from build123d import *

# Parameters (mm, degrees)
SKETCH_1_W      = 55
SKETCH_1_H      = 25
EXTRUDE_1_DEPTH = 1
FILLET_1_R      = 2


with BuildPart() as part:
    # Эскиз1 → Бобышка-Вытянуть1 (new body)
    with BuildSketch(Plane(origin=(0, 0, 0), x_dir=(1, 0, 0), z_dir=(0, 1, 0))):
        with Locations((-2.718269759, 0.212657213)):
            Rectangle(SKETCH_1_W, SKETCH_1_H)
        with BuildLine():
            Line((-18.218269759, 2.212657213), (-18.218269759, -1.787342787))
            ThreePointArc((-18.218269759, -1.787342787), (-20.218269759, -3.787342787), (-22.218269759, -1.787342787))
            Line((-22.218269759, -1.787342787), (-22.218269759, 2.212657213))
            ThreePointArc((-22.218269759, 2.212657213), (-20.218269759, 4.212657213), (-18.218269759, 2.212657213))
        make_face(mode=Mode.SUBTRACT)
        with BuildLine():
            Line((12.781730241, 2.212657213), (12.781730241, -1.787342787))
            ThreePointArc((12.781730241, -1.787342787), (14.781730241, -3.787342787), (16.781730241, -1.787342787))
            Line((16.781730241, -1.787342787), (16.781730241, 2.212657213))
            ThreePointArc((16.781730241, 2.212657213), (14.781730241, 4.212657213), (12.781730241, 2.212657213))
        make_face(mode=Mode.SUBTRACT)
    extrude(amount=EXTRUDE_1_DEPTH)

    # Скругление1
    fillet_1_edges = [part.edges().sort_by_distance(p)[0] for p in [
        (24.781730241, 0.5, 12.287342787),
        (-30.218269759, 0.5, 12.287342787),
        (-30.218269759, 0.5, -12.712657213),
        (24.781730241, 0.5, -12.712657213),
    ]]
    fillet(fillet_1_edges, radius=FILLET_1_R)


solid = part.part
Model file for the job. Use its own axes, mm. A direction names the side the tool comes from. Round coordinates to 2 decimals unless told otherwise and drop trailing zeros. Order: outer loops, then holes, each group sorted by start corner. A loop starts at its lowest first (then second) coordinate and runs counter-clockwise, first axis right, second up.
(1) Band-saw the part on A-A (y = 0.75). List the corners of the cut face in (x, z).
(2) 3-axis set-ups, long thin cutter, end or side, ignore diameter. For faces 5 (the face through (14.738, 0.493, 3.787)), 6 (the face through (24.782, 0.5, -0.1)): which of +Z, -Z, +X, -X, +Y, -Y reach the whole face in a straight line?
(3) Drill centre lines: line 1 (X direction, y = 0.3, z = -1.75); line 2 (X direction, y = 0.1, z = -2.75); line 3 (Z direction, x = -20, y = 0.2). Where is each one in solid material? Low to high.
(4) Band-saw the part on C-C (x = 15). List the corners of the cut face in (y, z).
(5) Pull direction X, two halves, no side cores. Call faces 1 (the face through (-30.218, 0.5, -0.1)), 2 (the face through (24.18, 0.51, -12.14)), 3 (the face through (-3, 0, 0)), 4 (the face through (16.782, 0.5, -0.2)): released by +X, released by -X, zero draft, split by the parting line, or undercut.
(6) Band-saw the part on D-D (z = -3.5). List the corners of the cut face in (x, y), then the cut area to 3 significant figures.
(7) Band-saw the part on B-B (z = 1). List the corners of the cut face in (x, y), then the cut area to 3 significant figures.
Verdict:
1. outline: (-30.22, -10.71) arc R2 ccw to (-28.22, -12.71) - (22.78, -12.71) arc R2 ccw to (24.78, -10.71) - (24.78, 10.29) arc R2 ccw to (22.78, 12.29) - (-28.22, 12.29) arc R2 ccw to (-30.22, 10.29) - close; hole (-22.22, -2.21) arc R2 ccw to (-18.22, -2.21) - (-18.22, 1.79) arc R2 ccw to (-22.22, 1.79) - close; hole (12.78, -2.21) arc R2 ccw to (16.78, -2.21) - (16.78, 1.79) arc R2 ccw to (12.78, 1.79) - close
2. face 5: +Y, -Y
2. face 6: +Z, -Z, +X, +Y, -Y
3. line 1: x = -30.22 to -22.22, -18.22 to 12.78, 16.78 to 24.78
3. line 2: x = -30.22 to -22.14, -18.29 to 12.86, 16.71 to 24.78
3. line 3: z = -12.71 to -4.2, 3.78 to 12.29
4. outline: (0, -12.71) - (1, -12.71) - (1, -4.2) - (0, -4.2) - close; (0, 3.78) - (1, 3.78) - (1, 12.29) - (0, 12.29) - close
5. face 1: released by -X
5. face 2: released by +X
5. face 3: zero draft
5. face 4: undercut
6. outline: (-30.22, 0) - (-21.75, 0) - (-21.75, 1) - (-30.22, 1) - close; (-18.69, 0) - (13.25, 0) - (13.25, 1) - (-18.69, 1) - close; (16.31, 0) - (24.78, 0) - (24.78, 1) - (16.31, 1) - close
6. area: 48.9 mm2
7. outline: (-30.22, 0) - (-22.22, 0) - (-22.22, 1) - (-30.22, 1) - close; (-18.22, 0) - (12.78, 0) - (12.78, 1) - (-18.22, 1) - close; (16.78, 0) - (24.78, 0) - (24.78, 1) - (16.78, 1) - close
7. area: 47.0 mm2
